```python
from build123d import *

# Parameters (mm, degrees)
F0_R       = 25.4
F1_DEPTH   = 7.62
F2_R       = 38.1
F1_FACE1_R = 25.4
F3_DEPTH   = 7.62
F4_R       = 2.54
F5_DEPTH   = 7.62
F7_D       = 5.4102
F7_DEPTH   = 8.89
F7_TIP     = 1.6253880605
F8_D       = 1.778


with BuildPart() as f1:
    # F0 (on Right) → F1 (new body)
    with BuildSketch(Plane.YZ):
        Circle(F0_R)
    extrude(amount=F1_DEPTH)

    # F2 (on face) + F1_face1 (on face) → F3 (join)
    with BuildSketch(Plane.YZ.offset(7.62)):
        Circle(F2_R)
    with BuildSketch(Plane(origin=(0, 0, 0), x_dir=(0, 1, 0), z_dir=(-1, 0, 0))):
        Circle(F1_FACE1_R)
    extrude(amount=F3_DEPTH, dir=(1, 0, 0))

    # F4 (on face) → F5 (cut)
    with BuildSketch(Plane.YZ.offset(15.24)):
        with Locations((0, 31.75)):
            Circle(F4_R)
        with Locations((27.4963065702, -15.875)):
            Circle(F4_R)
        with Locations((-27.4963065702, -15.875)):
            Circle(F4_R)
    extrude(amount=-F5_DEPTH, mode=Mode.SUBTRACT)

    # F7
    with Locations(Plane(origin=(0, 0, 0), x_dir=(0, -1, 0), z_dir=(-1, 0, 0))):
        with Locations((0, 0)):
            Hole(F7_D / 2, depth=F7_DEPTH)
            with Locations((0, 0, -(F7_DEPTH + F7_TIP / 2))):  # 118° drill point
                Cone(0, F7_D / 2, F7_TIP, mode=Mode.SUBTRACT)

    # F8 (through all)
    with Locations(Plane(origin=(0, 0, 0), x_dir=(0, -1, 0), z_dir=(-1, 0, 0))):
        with Locations((0, 0)):
            Hole(F8_D / 2)


solid = f1.part
```
Design review of the part built by this model. Coordinates are the model's own, in mm. A direction names the side the tool comes from. Round coordinates to 2 decimals unless told otherwise and drop trailing zeros. Order: outer loops, then holes, each group sorted by start corner. A loop starts at its lowest first (then second) coordinate and runs counter-clockwise, first axis right, second up. Notation, with made-up numbers: M 73,32.5 L 89,32.5 A20 ccw 89,66.5 Z; hole C 61.5,60.25 d6. An arc over 180 degrees is marked long. Put each result on its own line as item: value.
Q1. Consider section A-A (z = 0). State the section outline as (x, y) points.
Reported:
outline: M 0,-25.4 L 7.62,-25.4 L 7.62,-38.1 L 15.24,-38.1 L 15.24,-0.89 L 9.98,-0.89 L 8.89,-2.71 L 0,-2.71 Z; M 0,2.71 L 8.89,2.71 L 9.98,0.89 L 15.24,0.89 L 15.24,38.1 L 7.62,38.1 L 7.62,25.4 L 0,25.4 Z
Q2. Consider section B-B (y = 0). State the section outline as (x, z) points, and give its area (3 significant figures).
Reported:
outline: M 0,-25.4 L 7.62,-25.4 L 7.62,-38.1 L 15.24,-38.1 L 15.24,-0.89 L 9.98,-0.89 L 8.89,-2.71 L 0,-2.71 Z; M 0,2.71 L 8.89,2.71 L 9.98,0.89 L 15.24,0.89 L 15.24,29.21 L 7.62,29.21 L 7.62,25.4 L 0,25.4 Z; M 7.62,34.29 L 15.24,34.29 L 15.24,38.1 L 7.62,38.1 Z
area: 868 mm²
Q3. Draft analysis for pull direction Y (two halves, no side actions). For faces 3 (the face through (12.65, -0.19, -0.87)), 4 (the face through (7.62, 25, -8)), 5 (the face through (3.757, -5.506, -24.796)), state which applies: released by +Y, released by -Y, zero draft, split by the parting line, or undercut.
Reported:
face 3: undercut
face 4: zero draft
face 5: split by the parting line
Q4. To check wall thickness, follow line 1 (Z direction, x = 12.5, y = 0); line 2 (X direction, y = -4.5, z = 25.5); line 3 (Z direction, x = 6, y = 0). State the ranges of each line that lie inside material, in increasing order.
Reported:
line 1: -38.1 to -0.89, 0.89 to 29.21, 34.29 to 38.1
line 2: 7.62 to 15.24
line 3: -25.4 to -2.71, 2.71 to 25.4
Q5. Machinability: for faces 1 (the face through (11.48, -25.15, -16.85)), 2 (the face through (4.51, 2.58, 0.81)), which of the approach directions +Z, -Z, +X, -X, +Y, -Y give a long, thin tool a straight path to every point of the face, cutting with its end or side? Answer none if there is none.
Reported:
face 1: +X, -X
face 2: -X
Q6. Consider section D-D (x = 12.5). State the section outline as (y, z) points (3 decimals).
Reported:
outline: C 0,0 d76.2; hole C -27.496,-15.875 d5.08; hole C 0,31.75 d5.08; hole C 0,0 d1.778; hole C 27.496,-15.875 d5.08
Q7. Insertion check: pin 1 Ø2 at (y, z) = (-28, -8.5) entering from -X; pin 2 Ø4.5 at (y, z) = (27.5, -15.88) entering from -X; pin 3 Ø6 at (x, z) = (3, 11) entering from +Y; pin 4 Ø5 at (x, z) = (11, 19.5) entering from -Y. Each pin has a flat end and moves straight along its axis. Give the tip position at first contact, or say it passes through.
Reported:
pin 1: x = 7.62
pin 2: through
pin 3: y = 24.11
pin 4: y = -34.1
Q8. Consider section C-C (x = 2.75). State the section outline as (y, z) points, and give its area (3 significant figures).
Reported:
outline: C 0,0 d50.8; hole C 0,0 d5.41
area: 2,000 mm²
